Source: CAD feature listing. Evaluate the final solid. Frame: model axes, mm. Face numbers are marked on the shaded views. A direction names the side the tool comes from. Coordinates: 2 decimals unless noted, no trailing zeros. Loops run counter-clockwise (first coordinate to the right, second up) from the corner with the lowest first, then second, coordinate; pieces in that order, holes last. Notation, with made-up numbers: (49, 54) -> (72, 54) arc R14 ccw to (72, 61) -> close; hole circle Ø7 at (6.5, 2). An arc over 180 degrees is marked (long way). One line per question, with ' | ' between items. Start each with the question number.
```python
from build123d import *

# Parameters (mm, degrees)
SKETCH_1_R          = 3.8
EXTRUDE_1_DEPTH     = 4
SKETCH_2_W          = 9.2
SKETCH_2_H          = 9.2
EXTRUDE_2_DEPTH     = 0.5
FILLET_1_R          = 0.4
CUT_EXTRUDE_1_DEPTH = 4
CUT_EXTRUDE_2_DEPTH = 4
SKETCH_6_R          = 0.6
CUT_EXTRUDE_3_DEPTH = 8.636753289


with BuildPart() as part:
    # Эскиз1 → Бобышка-Вытянуть1 (new body)
    with BuildSketch(Plane.XY):
        Circle(SKETCH_1_R)
    extrude(amount=EXTRUDE_1_DEPTH)

    # Эскиз2 → Бобышка-Вытянуть2 (add)
    with BuildSketch(Plane(origin=(0, 0, 0), x_dir=(-1, 0, 0), z_dir=(0, 0, -1))):
        Rectangle(SKETCH_2_W, SKETCH_2_H)
    extrude(amount=EXTRUDE_2_DEPTH)

    # Скругление1
    fillet_1_edges = [part.edges().sort_by_distance(p)[0] for p in [
        (-3.8, 0, 4),
    ]]
    fillet(fillet_1_edges, radius=FILLET_1_R)

    # Эскиз3 → Вырез-Вытянуть1 (cut)
    with BuildSketch(Plane.XY.offset(4)):
        with BuildLine():
            Line((0.690974718, 1.998722557), (-0.494633441, 1.998722557))
            Line((-0.494633441, 1.998722557), (-0.967679121, 2.490729983))
            add(Edge.make_bspline(
                [(-0.967679121, 2.490729983), (-0.935743796, 2.513158419), (-0.873030504, 2.557202469), (-0.767844988, 2.603328706), (-0.657245689, 2.632663902), (-0.580977928, 2.635835465), (-0.542536801, 2.637434023)],
                knots=[0, 0, 0, 0, 1.020658978, 2.004328627, 2.994124718, 4, 4, 4, 4], degree=3))
            Line((-0.542536801, 2.637434023), (0.832688825, 2.637434023))
            Line((0.832688825, 2.637434023), (0.960431118, 2.624460196))
            Line((0.960431118, 2.624460196), (0.690974718, 1.998722557))
        make_face()
        with BuildLine():
            Line((0.783787478, 1.88096013), (1.080189518, 2.583542743))
            add(Edge.make_bspline(
                [(1.080189518, 2.583542743), (1.109972559, 2.568779947), (1.167520755, 2.540254577), (1.243334529, 2.484258604), (1.307175652, 2.420878144), (1.358952297, 2.349302652), (1.397359267, 2.268743846), (1.422764532, 2.180418501), (1.437519643, 2.084041158), (1.436172967, 2.017402915), (1.435472771, 1.98275477)],
                knots=[0, 0, 0, 0, 1.065948377, 2.059675685, 3.011626956, 3.94566096, 4.882319089, 5.862745984, 6.888747923, 8, 8, 8, 8], degree=3))
            Line((1.435472771, 1.98275477), (1.327690211, 0.277195558))
            Line((1.327690211, 0.277195558), (1.099151265, 0.106539838))
            Line((1.099151265, 0.106539838), (0.689976732, 0.433879465))
            Line((0.689976732, 0.433879465), (0.783787478, 1.88096013))
        make_face()
        with BuildLine():
            Line((0.639079412, -0.397443428), (1.085179451, -0.069105815))
            Line((1.085179451, -0.069105815), (1.293758665, -0.239761535))
            Line((1.293758665, -0.239761535), (1.192962011, -1.94432276))
            add(Edge.make_bspline(
                [(1.192962011, -1.94432276), (1.189491314, -1.97970738), (1.182773161, -2.048200607), (1.158848827, -2.146611673), (1.121568365, -2.235816828), (1.073168163, -2.317130934), (1.012395956, -2.389697225), (0.939872486, -2.454028672), (0.854949528, -2.509516087), (0.79219465, -2.538268676), (0.759835798, -2.553094627)],
                knots=[0, 0, 0, 0, 1.076355317, 2.083477241, 3.054916997, 3.995219207, 4.939832775, 5.910749548, 6.922701339, 8, 8, 8, 8], degree=3))
            Line((0.759835798, -2.553094627), (0.544270678, -1.848516041))
            Line((0.544270678, -1.848516041), (0.639079412, -0.397443428))
        make_face()
        with BuildLine():
            Line((-0.742134134, -1.961288534), (0.442476038, -1.961288534))
            Line((0.442476038, -1.961288534), (0.631095518, -2.593014093))
            Line((0.631095518, -2.593014093), (0.503353225, -2.6))
            Line((0.503353225, -2.6), (-0.869876427, -2.6))
            add(Edge.make_bspline(
                [(-0.869876427, -2.6), (-0.907959732, -2.598286355), (-0.982390401, -2.594937176), (-1.089588752, -2.568328401), (-1.188525215, -2.524510079), (-1.245499134, -2.481728782), (-1.274061027, -2.460281867)],
                knots=[0, 0, 0, 0, 1.046522757, 2.045342129, 3.020100256, 4, 4, 4, 4], degree=3))
            Line((-1.274061027, -2.460281867), (-0.742134134, -1.961288534))
        make_face()
        with BuildLine():
            Line((-0.827960987, -1.857497921), (-1.361883854, -2.364475147))
            add(Edge.make_bspline(
                [(-1.361883854, -2.364475147), (-1.382559986, -2.334279014), (-1.423593096, -2.274352853), (-1.460868358, -2.170727201), (-1.480865064, -2.060535537), (-1.47807852, -1.984986172), (-1.47665232, -1.946318734)],
                knots=[0, 0, 0, 0, 0.987067533, 1.958898816, 2.955330013, 4, 4, 4, 4], degree=3))
            Line((-1.47665232, -1.946318734), (-1.375855667, -0.240759522))
            Line((-1.375855667, -0.240759522), (-1.14432276, -0.069105815))
            Line((-1.14432276, -0.069105815), (-0.733152254, -0.398441415))
            Line((-0.733152254, -0.398441415), (-0.827960987, -1.857497921))
        make_face()
        with BuildLine():
            Line((-0.684250907, 0.434877451), (-1.131348934, 0.106539838))
            Line((-1.131348934, 0.106539838), (-1.339928147, 0.277195558))
            Line((-1.339928147, 0.277195558), (-1.232145587, 1.984750744))
            add(Edge.make_bspline(
                [(-1.232145587, 1.984750744), (-1.228217454, 2.022627769), (-1.220457829, 2.097449969), (-1.184381891, 2.204509013), (-1.134468518, 2.306511141), (-1.086053255, 2.365165228), (-1.061489867, 2.394923263)],
                knots=[0, 0, 0, 0, 1.007070456, 1.989364909, 2.979908279, 4, 4, 4, 4], degree=3))
            Line((-1.061489867, 2.394923263), (-0.590440161, 1.888944024))
            Line((-0.590440161, 1.888944024), (-0.684250907, 0.434877451))
        make_face()
        Polygon((-1.043526107, 0.018717012), (-0.598424054, 0.338072745), (0.593172025, 0.338072745), (0.997356625, 0.018717012), (0.553252558, -0.300638722), (-0.639341507, -0.300638722), align=None)
    extrude(amount=-CUT_EXTRUDE_1_DEPTH, mode=Mode.SUBTRACT)

    # Эскиз5 → Вырез-Вытянуть2 (cut)
    with BuildSketch(Plane.XY.offset(4)):
        with BuildLine():
            Line((1.080189518, 2.583542743), (0.960431118, 2.624460196))
            Line((0.960431118, 2.624460196), (0.832688825, 2.637434023))
            Line((0.832688825, 2.637434023), (-0.542536801, 2.637434023))
            add(Edge.make_bspline(
                [(-0.967679121, 2.490729983), (-0.935743796, 2.513158419), (-0.873030504, 2.557202469), (-0.767844988, 2.603328706), (-0.657245689, 2.632663902), (-0.580977928, 2.635835465), (-0.542536801, 2.637434023)],
                knots=[0, 0, 0, 0, 0.255164744, 0.501082157, 0.74853118, 1, 1, 1, 1], degree=3))
            Line((-0.967679121, 2.490729983), (-1.061489867, 2.394923263))
            add(Edge.make_bspline(
                [(-1.232145587, 1.984750744), (-1.228217454, 2.022627769), (-1.220457829, 2.097449969), (-1.184381891, 2.204509013), (-1.134468518, 2.306511141), (-1.086053255, 2.365165228), (-1.061489867, 2.394923263)],
                knots=[0, 0, 0, 0, 0.251767614, 0.497341227, 0.74497707, 1, 1, 1, 1], degree=3))
            Line((-1.232145587, 1.984750744), (-1.339928147, 0.277195558))
            Line((-1.339928147, 0.277195558), (-1.131348934, 0.106539838))
            Line((-1.131348934, 0.106539838), (-1.024891339, 0.01943817))
            Line((-1.024891339, 0.01943817), (-1.14432276, -0.069105815))
            Line((-1.14432276, -0.069105815), (-1.375855667, -0.240759522))
            Line((-1.375855667, -0.240759522), (-1.47665232, -1.946318734))
            add(Edge.make_bspline(
                [(-1.361883854, -2.364475147), (-1.382559986, -2.334279014), (-1.423593096, -2.274352853), (-1.460868358, -2.170727201), (-1.480865064, -2.060535537), (-1.47807852, -1.984986172), (-1.47665232, -1.946318734)],
                knots=[0, 0, 0, 0, 0.246766883, 0.489724704, 0.738832503, 1, 1, 1, 1], degree=3))
            Line((-1.361883854, -2.364475147), (-1.274061027, -2.460281867))
            add(Edge.make_bspline(
                [(-0.869876427, -2.6), (-0.907959732, -2.598286355), (-0.982390401, -2.594937176), (-1.089588752, -2.568328401), (-1.188525215, -2.524510079), (-1.245499134, -2.481728782), (-1.274061027, -2.460281867)],
                knots=[0, 0, 0, 0, 0.261630689, 0.511335532, 0.755025064, 1, 1, 1, 1], degree=3))
            Line((-0.869876427, -2.6), (0.503353225, -2.6))
            Line((0.503353225, -2.6), (0.631095518, -2.593014093))
            Line((0.631095518, -2.593014093), (0.759835798, -2.553094627))
            add(Edge.make_bspline(
                [(1.192962011, -1.94432276), (1.189491314, -1.97970738), (1.182773161, -2.048200607), (1.158848827, -2.146611673), (1.121568365, -2.235816828), (1.073168163, -2.317130934), (1.012395956, -2.389697225), (0.939872486, -2.454028672), (0.854949528, -2.509516087), (0.79219465, -2.538268676), (0.759835798, -2.553094627)],
                knots=[0, 0, 0, 0, 0.134544415, 0.260434655, 0.381864625, 0.499402401, 0.617479097, 0.738843694, 0.865337667, 1, 1, 1, 1], degree=3))
            Line((1.192962011, -1.94432276), (1.293758665, -0.239761535))
            Line((1.293758665, -0.239761535), (1.085179451, -0.069105815))
            Line((1.085179451, -0.069105815), (0.979606032, 0.017272437))
            Line((0.979606032, 0.017272437), (1.099151265, 0.106539838))
            Line((1.099151265, 0.106539838), (1.327690211, 0.277195558))
            Line((1.327690211, 0.277195558), (1.435472771, 1.98275477))
            add(Edge.make_bspline(
                [(1.080189518, 2.583542743), (1.109972559, 2.568779947), (1.167520755, 2.540254577), (1.243334529, 2.484258604), (1.307175652, 2.420878144), (1.358952297, 2.349302652), (1.397359267, 2.268743846), (1.422764532, 2.180418501), (1.437519643, 2.084041158), (1.436172967, 2.017402915), (1.435472771, 1.98275477)],
                knots=[0, 0, 0, 0, 0.133243547, 0.257459461, 0.376453369, 0.49320762, 0.610289886, 0.732843248, 0.86109349, 1, 1, 1, 1], degree=3))
        make_face()
    extrude(amount=-CUT_EXTRUDE_2_DEPTH, mode=Mode.SUBTRACT)

    # Эскиз6 → Вырез-Вытянуть3 (cut, through all)
    with BuildSketch(Plane.XY):
        Circle(SKETCH_6_R)
    extrude(amount=-CUT_EXTRUDE_3_DEPTH, mode=Mode.SUBTRACT)


solid = part.part
```
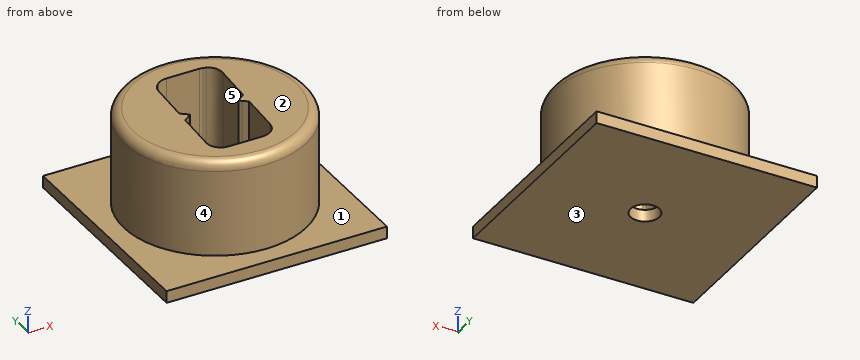
(1) Cut plane A-A, the plane x = 0. Return the cut outline in (y, z), and give its area (3 significant figures).
(2) Access query for the marked faces 1 and 2. Directions: +Z, -Z, +X, -X, +Y, -Y. A direction counts if a zero-diameter tool reaches every point of the face in a straight line with its end or side. Return the directions, or none.
(3) Contact query for flat-ended pins moving along their axis: pin 1 Ø1 at (x, z) = (2, 1.5) entering from +Y; pin 2 Ø1.5 at (x, z) = (3, 2.5) entering from -Y; pin 3 Ø1.5 at (x, z) = (0, 2) entering from -Y. Output: stop coordinate, or through.
(4) Draft query along X for the marked faces 3, 4 and 5. Return one class per face: pulls with the +X half, pulls with the -X half, needs draft (parallel to the pull), parting line crosses it, or undercut.
(5) Ray query, L1, parallel to Y at x = 0, z = -0.3; L2, parallel to X at y = -0.5, z = 1.15; L3, parallel to X at y = -2.5, z = 1.6. Return the intervals inside material, ascending.
Here are the results:
1) outline: (-4.6, -0.5) -> (-0.6, -0.5) -> (-0.6, 0) -> (-2.6, 0) -> (-2.6, 4) -> (-3.4, 4) arc R0.4 ccw to (-3.8, 3.6) -> (-3.8, 0) -> (-4.6, 0) -> close; (0.6, -0.5) -> (4.6, -0.5) -> (4.6, 0) -> (3.8, 0) -> (3.8, 3.6) arc R0.4 ccw to (3.4, 4) -> (2.64, 4) -> (2.64, 0) -> (0.6, 0) -> close | area: 13.4 mm2
2) face 1: +Z | face 2: +Z, +X, -X, +Y, -Y
3) pin 1: stops at y = 3.49 | pin 2: stops at y = -3.06 | pin 3: stops at y = -3.8
4) face 3: needs draft | face 4: parting line crosses it | face 5: undercut
5) L1: y = -4.6 to -0.6, 0.6 to 4.6 | L2: x = -3.77 to -1.39, 1.28 to 3.77 | L3: x = -2.86 to -1.22, 0.87 to 2.86
